```python
from build123d import *

# Parameters (mm, degrees)
SKETCH2_R          = 3
CUT_EXTRUDE1_DEPTH = 103.225241501


with BuildPart() as part:
    # Sketch1 → Revolve1 (revolve)
    with BuildSketch(Plane(origin=(0, 0, 0), x_dir=(0, 0, -1), z_dir=(1, 0, 0))):
        with BuildLine():
            Line((-43.75, 55), (-45, 55))
            Line((-45, 55), (-45, -55))
            ThreePointArc((-45, -55), (-42.071067812, -62.071067812), (-35, -65))
            Line((-35, -65), (-15, -65))
            ThreePointArc((-15, -65), (-7.928932188, -67.928932188), (-5, -75))
            Line((-5, -75), (-5, -80))
            Line((-5, -80), (-4, -80))
            Line((-4, -80), (-4, -70))
            ThreePointArc((-4, -70), (-6.928932188, -62.928932188), (-14, -60))
            Line((-14, -60), (-30, -60))
            ThreePointArc((-30, -60), (-37.071067812, -57.071067812), (-40, -50))
            Line((-40, -50), (-40, -18.031088913))
            Line((-40, -18.031088913), (-38.25, -15))
            Line((-38.25, -15), (-40.75, -15))
            Line((-40.75, -15), (-40.75, 28))
            Line((-40.75, 28), (-39.75, 30))
            Line((-39.75, 30), (-42.25, 30))
            Line((-42.25, 30), (-42.25, 50))
            Line((-42.25, 50), (-43.75, 50))
            Line((-43.75, 50), (-43.75, 55))
        make_face()
    revolve(axis=Axis((0, 48.80804048, 0), (0, -1, 0)))

    # Sketch2 → Cut-Extrude1 (cut, through all)
    with BuildSketch(Plane.XY):
        with Locations((0, -10)):
            Circle(SKETCH2_R)
    extrude(amount=-CUT_EXTRUDE1_DEPTH, mode=Mode.SUBTRACT)


solid = part.part
```
The listing builds one solid part. Answer for the finished solid, in the listing's coordinates (mm). A direction names the side the tool comes from. Give positions to 0.01 mm unless a question says otherwise; leave off trailing zeros. Loops run counter-clockwise (first coordinate to the right, second up) from the corner with the lowest first, then second, coordinate; pieces in that order, holes last. Notation, with made-up numbers: (-0.5, -29.5) - (20.5, -29.5) arc R21 ccw to (20.5, -0.5) - close; hole circle Ø4 at (34.5, -5.75). An arc over 180 degrees is marked (long way). Answer as CSV lines item,"result". Start each with the question number.
Item 1: Find the intervals of material crossed by line 1 (X direction, y = -30, z = 0); line 2 (X direction, y = -11, z = 0); line 3 (Z direction, x = 0, y = 53.6), in increasing order. Write a range as from..to.
Item 2: A cutting plane is placed at B-B on x = 0. Count the separate pieces of the cut face and the enclosed holes in it, then the cut area to 3 significant figures.
Item 3: A cutting plane is placed at C-C on y = 23. Determine the outline of the cut face in (x, z), then the cut area to 3 significant figures.
Item 4: For faces 4 (the face through (13, -60, -6)), 5 (the face through (0, -7, -43)), 6 (the face through (15.61, 6.8, 37.64)), 7 (the face through (3.905, -74.93, -0.867)), determine the directions among +Z, -Z, +X, -X, +Y, -Y from which every point of the face is accessible in a straight line to the end or side of a thin tool.
Item 5: Each of these flat-tipped pins is pushed along its axis until it touches: pin 1 (6 mm diameter, centred on x = -23.5, z = 28, fed in from +Y); pin 2 (12 mm diameter, centred on y = -54.5, z = 20.5, fed in from +X); pin 3 (3 mm diameter, centred on x = 29, z = -18.5, fed in from -Y). Where does it stop, or does it pass through?
Item 6: The mould has two halves that part along Z. Classify faces 1 (the face through (7, -65, 15)), 2 (the face through (4.88, -77.54, -1.08)), 3 (the face through (-36, 50, 23)): +Z half, -Z half, draft (parallel to the pull), parting line (faces both ways), or undercut.
Item 7: A cutting plane is placed at A-A on y = -38.5. Determine the outline of the cut face in (x, z), then the cut area to 3 significant figures.
Item 8: A cutting plane is placed at D-D on y = -10. Determine the outline of the cut face in (x, z), then the cut area to 3 significant figures.
Found:
1,line 1,"x = -45..-40, 40..45"
1,line 2,"x = -45..-40.75, 40.75..45"
1,line 3,"z = -45..-43.75, 43.75..45"
2,separate pieces,"3"
2,enclosed holes,"0"
2,area,"1,380 mm^2"
3,outline,"circle Ø90 at (0, 0); hole circle Ø81.5 at (0, 0)"
3,area,"1,140 mm^2"
4,face 4,"+Y"
4,face 5,"-Z"
4,face 6,"none"
4,face 7,"+Y, -Y"
5,pin 1,"stops at y = -15"
5,pin 2,"stops at x = 42.6"
5,pin 3,"stops at y = -65"
6,face 1,"draft"
6,face 2,"parting line"
6,face 3,"undercut"
7,outline,"circle Ø90 at (0, 0); hole circle Ø80 at (0, 0)"
7,area,"1,340 mm^2"
8,outline,"(-3, -44.9) - (-3, -40.64) arc R40.75 cw (long way) to (3, -40.64) - (3, -44.9) arc R45 ccw (long way) to start"
8,area,"1,120 mm^2"
